The drawing under review shows one solid part. Ordinate dimensions are in mm from its lowest x, y, z. A direction names the side the tool comes from. Round coordinates to 2 decimals unless told otherwise and drop trailing zeros. Order: outer loops, then holes, each group sorted by start corner. A loop starts at its lowest first (then second) coordinate and runs counter-clockwise, first axis right, second up. Notation, with made-up numbers: M -25.75,9 L 26.25,9 A31 ccw 26.25,36 Z; hole C 11,-3.75 d2. An arc over 180 degrees is marked long. Use a Markdown table: item, result.
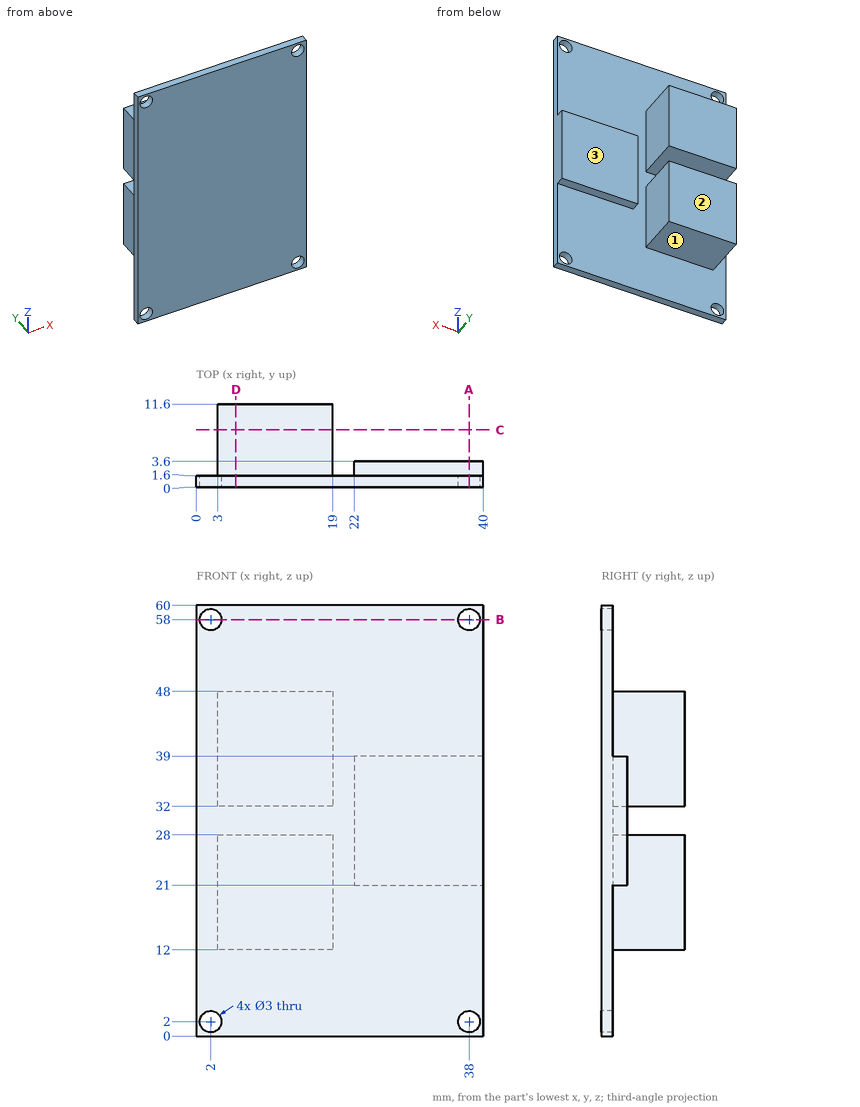
Q1. Add section B-B (z = 58). Write out the cut boundary in (x, y), then the cut area to 3 significant figures.
Determined:
| item | result |
|---|---|
| outline | M 0,0 L 0.5,0 L 0.5,1.6 L 0,1.6 Z; M 3.5,0 L 36.5,0 L 36.5,1.6 L 3.5,1.6 Z; M 39.5,0 L 40,0 L 40,1.6 L 39.5,1.6 Z |
| area | 54.4 mm^2 |
Q2. Add section D-D (x = 5.5). Write out the cut boundary in (y, z).
Determined:
| item | result |
|---|---|
| outline | M 0,0 L 1.6,0 L 1.6,12 L 11.6,12 L 11.6,28 L 1.6,28 L 1.6,32 L 11.6,32 L 11.6,48 L 1.6,48 L 1.6,60 L 0,60 Z |
Q3. Wall thickness on line 1 along Z through (x, y) = (38, 0.6); line 2 along X through (y, z) = (2, 35); line 3 along X through (y, z) = (5, 20): over which ranges is each line inside the solid? List them lowest first. Write a range as [from, to].
Determined:
| item | result |
|---|---|
| line 1 | z = [0, 0.5], [3.5, 56.5], [59.5, 60] |
| line 2 | x = [3, 19], [22, 40] |
| line 3 | x = [3, 19] |
Q4. Add section C-C (y = 8). Write out the cut boundary in (x, z), then the cut area to 3 significant figures.
Determined:
| item | result |
|---|---|
| outline | M 3,12 L 19,12 L 19,28 L 3,28 Z; M 3,32 L 19,32 L 19,48 L 3,48 Z |
| area | 512 mm^2 |
Q5. Add section A-A (x = 38). Write out the cut boundary in (y, z), then the cut area to 3 significant figures.
Determined:
| item | result |
|---|---|
| outline | M 0,0 L 1.6,0 L 1.6,0.5 L 0,0.5 Z; M 0,3.5 L 1.6,3.5 L 1.6,21 L 3.6,21 L 3.6,39 L 1.6,39 L 1.6,56.5 L 0,56.5 Z; M 0,59.5 L 1.6,59.5 L 1.6,60 L 0,60 Z |
| area | 122 mm^2 |
Q6. Machinability: for the marked faces 1, 2 and 3, which of the approach directions +Z, -Z, +X, -X, +Y, -Y give a long, thin tool a straight path to every point of the face, cutting with its end or side? Answer none if there is none.
Determined:
| item | result |
|---|---|
| face 1 | -Z, +X, -X, +Y |
| face 2 | +Z, -Z, +X, -X, +Y |
| face 3 | +Z, -Z, +X, +Y |
Q7. Clearance check with flat-ended pins moving along their axes: pin 1 (4 mm diameter, centred on y = 8, z = 33.5, fed in from +X); pin 2 (3 mm diameter, centred on y = 7, z = 19.5, fed in from -X); pin 3 (3 mm diameter, centred on x = 11.5, y = 4.5, fed in from +Z); pin 4 (5 mm diameter, centred on x = 4.5, z = 20, fed in from -Y). State where each tip first meets the part, or that it passes through.
Determined:
| item | result |
|---|---|
| pin 1 | stops at x = 19 |
| pin 2 | stops at x = 3 |
| pin 3 | stops at z = 48 |
| pin 4 | stops at y = 0 |
